Work out the finished part from the listing and answer in its coordinate system (mm). Face numbers are marked on the shaded views. A direction names the side the tool comes from. Give positions to 0.01 mm unless a question says otherwise; leave off trailing zeros. Loops run counter-clockwise (first coordinate to the right, second up) from the corner with the lowest first, then second, coordinate; pieces in that order, holes last. Notation, with made-up numbers: (38, 38) - (65, 38) arc R32 cw to (65, 70) - close; hole circle Ø5 at (55, 79). An arc over 180 degrees is marked (long way). Use one line per item in the form item = value. Start each with the question number.
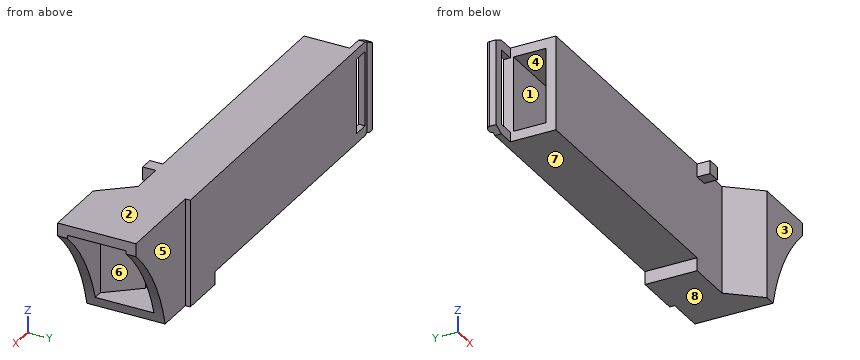
from build123d import *

# Parameters (mm, degrees)
RESSALTO_EXTRUS_O1_DEPTH   = 16.5
CORTE_EXTRUS_O3_DEPTH      = 1
CORTE_EXTRUS_O3_DEPTH_BACK = 13.75
CASCA1_T                   = -1.5
CORTE_EXTRUS_O2_DEPTH      = 13.75
ESBO_O6_W                  = 60.936281692
ESBO_O6_H                  = 31.71485299
CORTE_EXTRUS_O4_DEPTH      = 3
CORTE_EXTRUS_O4_DEPTH_BACK = 15.5
RESSALTO_EXTRUS_O2_DEPTH   = 14.5
ESBO_O8_W                  = 2.5
ESBO_O8_H                  = 11.5
CORTE_EXTRUS_O5_DEPTH      = 10
ESBO_O9_W                  = 2
ESBO_O9_H                  = 2
RESSALTO_EXTRUS_O3_DEPTH   = 2
ESBO_O10_W                 = 2
ESBO_O10_H                 = 2
RESSALTO_EXTRUS_O4_DEPTH   = 8


with BuildPart() as part:
    # Esboço1 → Ressalto-extrusão1 (new body)
    with BuildSketch(Plane.XY):
        with BuildLine():
            Line((9.53089658, 0), (70, 0))
            Line((70, 0), (70, -0.75))
            Line((70, -0.75), (84, -0.75))
            Line((84, -0.75), (84, -12.75))
            Line((84, -12.75), (74, -12.75))
            Line((74, -12.75), (70, -8))
            Line((70, -8), (6.002125959, -8))
            Line((6.002125959, -8), (5.638155725, -9))
            Line((5.638155725, -9), (0, -6.94787914))
            Line((0, -6.94787914), (0.133970372, -6.579798567))
            ThreePointArc((0.133970372, -6.579798567), (3.795132217, -1.808479557), (9.53089658, 0))
        make_face()
    extrude(amount=RESSALTO_EXTRUS_O1_DEPTH)

    # Esboço5 → Corte-extrusão3 (cut, two sides)
    with BuildSketch(Plane.XZ.offset(12.75)) as corte_extrus_o3_sk:
        Polygon((0, 0), (65, 0), (63, 2), (0, 2), align=None)
    extrude(amount=CORTE_EXTRUS_O3_DEPTH, mode=Mode.SUBTRACT)
    extrude(corte_extrus_o3_sk.sketch, amount=-CORTE_EXTRUS_O3_DEPTH_BACK, mode=Mode.SUBTRACT)

    # Casca1
    casca1_openings = [part.faces().sort_by_distance(p)[0] for p in [
        (84, -6.75, 8.25),
        (2.819077862, -7.97393957, 9.25),
    ]]
    offset(amount=CASCA1_T, openings=casca1_openings, kind=Kind.INTERSECTION)

    # Esboço4 → Corte-extrusão2 (cut, through all)
    with BuildSketch(Plane.XZ.offset(12.75)):
        with BuildLine():
            Line((75.737834478, 0), (84, 0))
            Line((84, 0), (84, 14.5))
            ThreePointArc((84, 14.5), (78.803340396, 7.8571705), (75.737834478, 0))
        make_face()
    extrude(amount=-CORTE_EXTRUS_O2_DEPTH, mode=Mode.SUBTRACT)

    # Esboço6 → Corte-extrusão4 (cut, two sides)
    with BuildSketch(Plane(origin=(0, 0, 2), x_dir=(-1, 0, 0), z_dir=(0, 0, -1))) as corte_extrus_o4_sk:
        with Locations((7.468140846, -5.914756455)):
            Rectangle(ESBO_O6_W, ESBO_O6_H)
    extrude(amount=CORTE_EXTRUS_O4_DEPTH, mode=Mode.SUBTRACT)
    extrude(corte_extrus_o4_sk.sketch, amount=-CORTE_EXTRUS_O4_DEPTH_BACK, mode=Mode.SUBTRACT)

    # Esboço7 → Ressalto-extrusão2 (add)
    with BuildSketch(Plane.XY.offset(16.5)):
        with BuildLine():
            Line((23, 0), (20, 0))
            ThreePointArc((20, 0), (19.5, 0.5), (19, 0))
            Line((19, 0), (19, -1))
            Line((19, -1), (23, -1))
            Line((23, -1), (23, 0))
        make_face()
    extrude(amount=-RESSALTO_EXTRUS_O2_DEPTH)

    # Esboço8 → Corte-extrusão5 (cut)
    with BuildSketch(Plane.XZ.offset(1)):
        with Locations((21.75, 9.25)):
            Rectangle(ESBO_O8_W, ESBO_O8_H)
        Polygon((20.5, 16.5), (19, 16.5), (19, 15.8), align=None)
        Polygon((19, 2.7), (20.5, 2), (19, 2), align=None)
    extrude(amount=-CORTE_EXTRUS_O5_DEPTH, mode=Mode.SUBTRACT)

    # Esboço9 → Ressalto-extrusão3 (add)
    with BuildSketch(Plane.XZ.offset(8)):
        with Locations((64, 15.5)):
            Rectangle(ESBO_O9_W, ESBO_O9_H)
    extrude(amount=RESSALTO_EXTRUS_O3_DEPTH)

    # Esboço10 → Ressalto-extrusão4 (add)
    with BuildSketch(Plane.XZ.offset(8)):
        with Locations((64, 1)):
            Rectangle(ESBO_O10_W, ESBO_O10_H)
    extrude(amount=-RESSALTO_EXTRUS_O4_DEPTH)


solid = part.part
1) A cutting plane is placed at B-B (y = -3.25). Give the vertices of the cut face in (x, z).
2) Flat-ended cylindrical pins translate along their axes: pin 1 Ø0.6 at (x, z) = (64, 16) entering from -Y; pin 2 Ø0.8 at (y, z) = (-2, 5.5) entering from -X; pin 3 Ø6 at (y, z) = (-9.5, 8.5) entering from +X; pin 4 Ø8 at (x, z) = (71, 2.5) entering from -Y. Find the tip coordinate at first contact, or state that the pin passes through.
3) A cutting plane is placed at C-C (z = 7). Give the vertices of the cut face in (x, y), plus the area to 3 significant figures.
4) A tool of negligible diameter and unlimited length cuts with its end or side. For the marked faces 4, 5, 6, 7 and 8, from which of +Z, -Z, +X, -X, +Y, -Y can it reach the whole face along a straight path? Write none if from no direction.
5) Determine the mould class of the marked faces 1, 2 and 3 for opening direction Z: released by +Z, released by -Z, zero draft, split by the parting line, or undercut.
6) Find the intervals of material crossed by probe 1 along Y at (x, z) = (38, 13.5); probe 2 along X at (y, z) = (-0.5, 14); probe 3 along Z at (x, y) = (27.5, -7.5), in increasing order.
7) A cutting plane is placed at D-D (x = 77). Give the vertices of the cut face in (y, z).
8) A cutting plane is placed at A-A (x = 55). Give the vertices of the cut face in (y, z).
Answer sheet:
q1.outline = (23, 2) - (63, 2) - (63, 0) - (75.74, 0) arc R29 cw to (76.13, 1.5) - (65.62, 1.5) - (63.62, 3.5) - (23, 3.5) - close; (23, 15) - (84, 15) - (84, 16.5) - (23, 16.5) - close
q2.pin_1 = -10
q2.pin_2 = 68.5
q2.pin_3 = 80.83
q2.pin_4 = -12.75
q3.outline = (19, -1) - (20.5, -1) - (20.5, 0) - (20, 0) arc R0.5 ccw to (19, 0) - close; (23, -8) - (70, -8) - (74, -12.75) - (78.33, -12.75) - (78.33, -11.25) - (74.7, -11.25) - (70.7, -6.5) - (23, -6.5) - close; (23, -1.5) - (68.5, -1.5) - (68.5, -2.25) - (78.33, -2.25) - (78.33, -0.75) - (70, -0.75) - (70, 0) - (23, 0) - close
q3.area = 172 mm²
q4.face_4 = none
q4.face_5 = +Z, -Z, +X, +Y
q4.face_6 = +X
q4.face_7 = -Z, -X, +Y, -Y
q4.face_8 = -Z, +X, -X, +Y, -Y
q5.face_1 = undercut
q5.face_2 = released by +Z
q5.face_3 = zero draft
q6.probe_1 = -8 to -6.5, -1.5 to 0
q6.probe_2 = 19 to 20.5, 23 to 70
q6.probe_3 = 2 to 16.5
q7.outline = (-12.75, 4.08) - (-11.25, 4.08) - (-11.25, 15) - (-2.25, 15) - (-2.25, 4.08) - (-0.75, 4.08) - (-0.75, 16.5) - (-12.75, 16.5) - close
q8.outline = (-8, 2) - (0, 2) - (0, 16.5) - (-8, 16.5) - close; hole (-6.5, 3.5) - (-1.5, 3.5) - (-1.5, 15) - (-6.5, 15) - close
